Geometry: final body of the model. Coordinates: model frame, mm. Face numbers are marked on the shaded views. Coordinates: 2 decimals unless noted, no trailing zeros. Write each loop counter-clockwise with the first axis right and the second up, starting at its lowest first coordinate (ties: lowest second). Pieces come first, ordered by that corner, then holes. Notation, with made-up numbers: (32.25, 77) - (54.25, 77) arc R19 ccw to (54.25, 103) - close; hole circle Ø10 at (33, 38). An arc over 180 degrees is marked (long way). Answer as a JSON object with one key per item and string values. Group by question number.
Item 1: First-contact query: pin 1 Ø2 at (x, z) = (39.5, 16) entering from -Y; pin 2 Ø1 at (x, z) = (31.5, 19.5) entering from -Y; pin 3 Ø6 at (y, z) = (9, 12.5) entering from -X. Flat tips, straight axial feed; report the tip coordinate or a pass-through.
Item 2: Section C-C on z = 12.75. Return loops of the section in (x, y).
Item 3: Section D-D on y = 35. Return loops of the section in (x, z), and give its area (3 significant figures).
Item 4: Section B-B on y = -2.5. Return loops of the section in (x, z).
Item 5: Section A-A on x = -16.5. Return loops of the section in (y, z), and give its area (3 significant figures).
Item 6: Line query: line 1 along Y through (x, z) = (5, 14.5); line 2 along Y through (x, z) = (8, 16.75); line 3 along X through (y, z) = (1, 9). Output: solid intervals per line, ascending. Write a range as from..to.
Item 7: Mould query, pull axis Y, two halves, no side actions, for the marked faces 1, 2 and 3. Classes: pulls with the +Y half, pulls with the -Y half, needs draft (parallel to the pull), parting line crosses it, or undercut.
```python
from build123d import *

# Parameters (mm, degrees)
F0_R     = 15.043231
F0_R_2   = 29.884634
F1_DEPTH = 25.4


with BuildPart() as f1:
    # F0 (on Top) → F1 (new body)
    with BuildSketch(Plane.XY):
        with BuildLine():
            ThreePointArc((57.019541, 0.869514), (-0.43477, 57.024513), (-57.02617, 0))
            Line((-57.02617, 0), (-19.565552, -143.03863))
            ThreePointArc((-19.565552, -143.03863), (20.135156, -178.433137), (57.019541, -140.112653))
            Line((57.019541, -140.112653), (57.019541, 0.869514))
        make_face()
        with Locations((18.6711, -140.112653)):
            Circle(F0_R, mode=Mode.SUBTRACT)
        Circle(F0_R_2, mode=Mode.SUBTRACT)
    extrude(amount=F1_DEPTH)


solid = f1.part
```
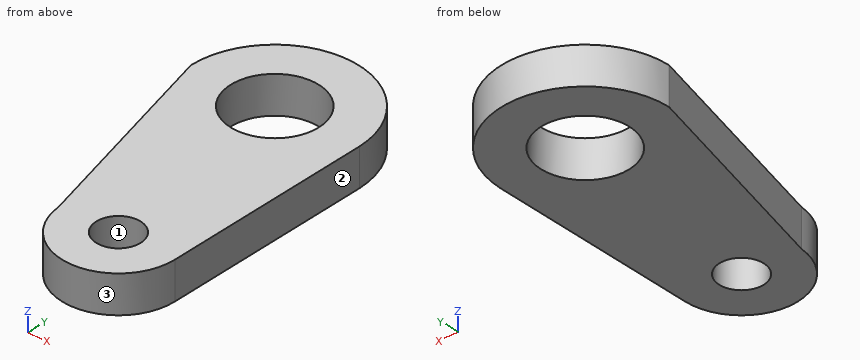
Checks:
{
 "1": {"pin 1": "y = -172.94", "pin 2": "y = -176.43", "pin 3": "x = -56.71"},
 "2": {"outline": "(-57.03, 0) - (-19.57, -143.04) arc R38.35 ccw to (57.02, -140.11) - (57.02, 0.87) arc R57.03 ccw to start; hole circle Ø59.77 at (0, 0); hole circle Ø30.09 at (18.67, -140.11)"},
 "3": {"outline": "(-45.02, 0) - (45.02, 0) - (45.02, 25.4) - (-45.02, 25.4) - close", "area": "2,290 mm^2"},
 "4": {"outline": "(-56.37, 0) - (-29.78, 0) - (-29.78, 25.4) - (-56.37, 25.4) - close; (29.78, 0) - (57.02, 0) - (57.02, 25.4) - (29.78, 25.4) - close"},
 "5": {"outline": "(-155.4, 0) - (-24.92, 0) - (-24.92, 25.4) - (-155.4, 25.4) - close; (24.92, 0) - (54.59, 0) - (54.59, 25.4) - (24.92, 25.4) - close", "area": "4,070 mm^2"},
 "6": {"line 1": "-175.94..-146.39, -133.84..-29.46, 29.46..56.81", "line 2": "-176.95..-150.72, -129.51..-28.79, 28.79..56.46", "line 3": "-57.02..-29.87, 29.87..57.02"},
 "7": {"face 1": "undercut", "face 2": "needs draft", "face 3": "pulls with the -Y half"}
}
